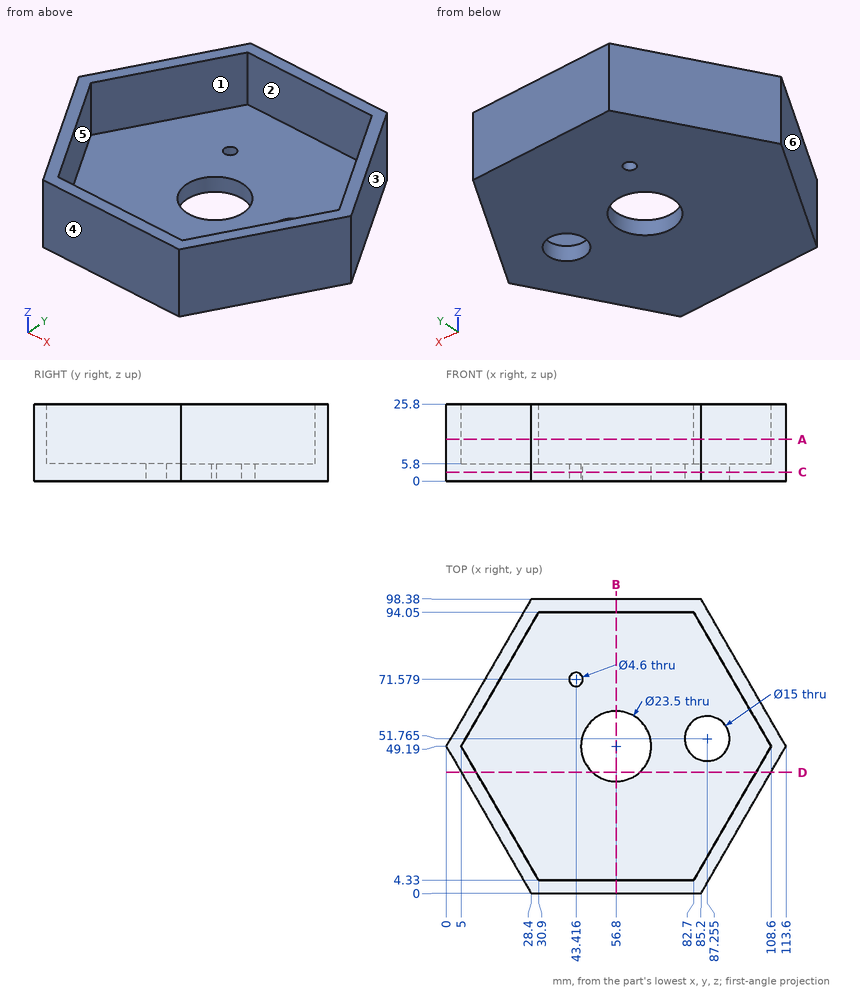
Could you check a few things on this drawing? It's one solid part, dimensions in mm from its lowest x, y, z. A direction names the side the tool comes from. Round coordinates to 2 decimals unless told otherwise and drop trailing zeros. Order: outer loops, then holes, each group sorted by start corner. A loop starts at its lowest first (then second) coordinate and runs counter-clockwise, first axis right, second up. Notation, with made-up numbers: M 51,42 L 82,42 A15 ccw 82,55 Z; hole C 35,-14 d11. An arc over 180 degrees is marked long. One line per item, written item: value.
(1) Imagine slicing it at D-D (y = 40.5). Write out the boundary of the cut face in (x, z), and give its area (3 significant figures).
Ans:
outline: M 5.02,0 L 48.89,0 L 48.89,5.8 L 10.02,5.8 L 10.02,25.8 L 5.02,25.8 Z; M 64.71,0 L 108.58,0 L 108.58,25.8 L 103.58,25.8 L 103.58,5.8 L 64.71,5.8 Z
area: 709 mm^2
(2) Imagine slicing it at C-C (z = 3). Count the separate pieces of the cut face and the enclosed holes in it.
Ans:
separate pieces: 1
enclosed holes: 3
(3) Which directions (+Z, -Z, +X, -X, +Y, -Y) give clear straight access to the entire face, cutting with the end or side of a thin tool? Please do the marked faces 5 and 6.
Ans:
face 5: +Z
face 6: +Z, -Z, -X, -Y
(4) Imagine slicing it at B-B (x = 56.8). Write out the boundary of the cut face in (y, z).
Ans:
outline: M 0,0 L 37.44,0 L 37.44,5.8 L 4.33,5.8 L 4.33,25.8 L 0,25.8 Z; M 60.94,0 L 98.38,0 L 98.38,25.8 L 94.05,25.8 L 94.05,5.8 L 60.94,5.8 Z
(5) Imagine slicing it at A-A (z = 14). Write out the boundary of the cut face in (x, y).
Ans:
outline: M 0,49.19 L 28.4,0 L 85.2,0 L 113.6,49.19 L 85.2,98.38 L 28.4,98.38 Z; hole M 5,49.19 L 30.9,4.33 L 82.7,4.33 L 108.6,49.19 L 82.7,94.05 L 30.9,94.05 Z
(6) If we mould it in two halves opening along X, with no side actions, what happens to the marked faces 1, 2, 3 and 4? For each: released by +X, released by -X, zero draft, split by the parting line, or undercut.
Ans:
face 1: undercut
face 2: undercut
face 3: released by +X
face 4: zero draft
(7) I'm going to push flat-ended pins straight in: P1, Ø8, axis at y = 52.5, z = 19.5, coming from the -X side; P2, Ø21, axis at x = 56.8, y = 49.19, coming from the +Z side; P3, Ø10, axis at y = 72.5, z = 20.5, coming from the +X side; P4, Ø4, axis at y = 74.5, z = 8, coming from the -X side. Where does each tip first touch, or does it pass through?
Ans:
P1: stops at x = 0
P2: passes through
P3: stops at x = 103.03
P4: stops at x = 13.46
(8) I need wall thicknesses on line 1 along Y through (x, z) = (34, 24.25); line 2 along Y through (x, z) = (56.8, 2.8); line 3 along Z through (x, y) = (31.5, 50). Which ranges of each line are inside material? Lowest first, please. Write a range as from..to.
Ans:
line 1: y = 0..4.33, 94.05..98.38
line 2: y = 0..37.44, 60.94..98.38
line 3: z = 0..5.8
